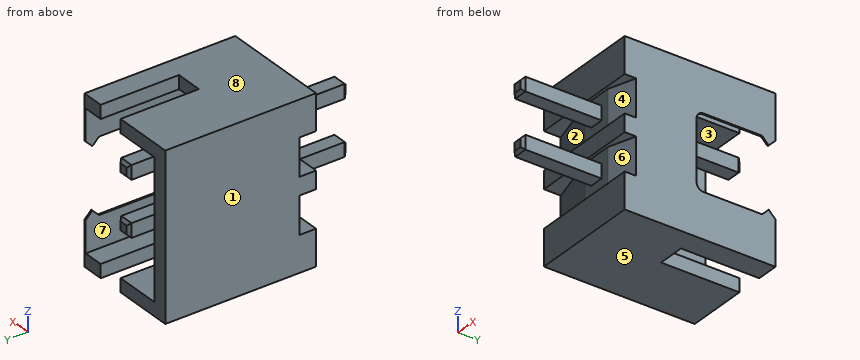
```python
from build123d import *

# Parameters (mm, degrees)
SKETCH1_W           = 6.8453
SKETCH1_H           = 7.4295
BOSS_EXTRUDE1_DEPTH = 5
SKETCH2_W           = 5.8039
SKETCH2_H           = 0.127
CUT_EXTRUDE1_DEPTH  = 5.7277
CUT_EXTRUDE2_DEPTH  = 1.6891
CUT_EXTRUDE3_DEPTH  = 1.6891
SKETCH5_W           = 5
SKETCH5_H           = 4.1148
BOSS_EXTRUDE2_DEPTH = 0.127
SKETCH6_W           = 3.3147
SKETCH6_H           = 0.127
CUT_EXTRUDE4_DEPTH  = 6
CUT_EXTRUDE5_DEPTH  = 1.6891
CUT_EXTRUDE6_DEPTH  = 1.6891
SKETCH9_W           = 5
SKETCH9_H           = 1.6256
BOSS_EXTRUDE3_DEPTH = 0.127
SKETCH10_W          = 4.2672
SKETCH10_H          = 6.2103
CUT_EXTRUDE7_DEPTH  = 5.1308
CUT_EXTRUDE8_DEPTH  = 1.0724
SKETCH12_W          = 1.2319
SKETCH12_H          = 3.556
CUT_EXTRUDE9_DEPTH  = 1.6096
SKETCH13_W          = 1.2319
SKETCH13_H          = 3.556
CUT_EXTRUDE10_DEPTH = 8.4295
SKETCH14_W          = 0.635
SKETCH14_H          = 0.635
BOSS_EXTRUDE4_DEPTH = 3.5814
SKETCH15_W          = 0.635
SKETCH15_H          = 0.635
BOSS_EXTRUDE5_DEPTH = 3.5814
SKETCH16_W          = 0.635
SKETCH16_H          = 0.635
BOSS_EXTRUDE6_DEPTH = 4.7625
SKETCH17_W          = 0.635
SKETCH17_H          = 0.635
BOSS_EXTRUDE7_DEPTH = 4.7625
DRAFT1_ANGLE        = 45
DRAFT2_ANGLE        = 45
CHAMFER1_SIZE       = 0.127
FILLET1_R           = 0.3175


with BuildPart() as part:
    # Sketch1 → Boss-Extrude1 (new body)
    with BuildSketch(Plane(origin=(-5.7277, 0, 0), x_dir=(0, -1, 0), z_dir=(-1, 0, 0))):
        with Locations((-3.42265, -3.71475)):
            Rectangle(SKETCH1_W, SKETCH1_H)
    extrude(amount=-BOSS_EXTRUDE1_DEPTH)

    # Sketch2 → Cut-Extrude1 (cut)
    with BuildSketch(Plane.ZY.offset(5.7277)):
        with Locations((-4.52755, 0.0635)):
            Rectangle(SKETCH2_W, SKETCH2_H)
    extrude(amount=-CUT_EXTRUDE1_DEPTH, mode=Mode.SUBTRACT)

    # Sketch3 → Cut-Extrude2 (cut)
    with BuildSketch(Plane.XY.offset(-1.6256)):
        Polygon((-5.7277, 0.127), (-3.3477, 0.127), (-5.7277, 0.762), align=None)
    extrude(amount=-CUT_EXTRUDE2_DEPTH, mode=Mode.SUBTRACT)

    # Sketch4 → Cut-Extrude3 (cut)
    with BuildSketch(Plane.XY.offset(-1.6256)):
        Polygon((-1.94, 0.127), (0, 0.127), (0, 0.762), align=None)
    extrude(amount=-CUT_EXTRUDE3_DEPTH, mode=Mode.SUBTRACT)

    # Sketch5 → Boss-Extrude2 (add)
    with BuildSketch(Plane.XZ.offset(-0.127)):
        with Locations((-3.2277, -5.3721)):
            Rectangle(SKETCH5_W, SKETCH5_H)
    extrude(amount=BOSS_EXTRUDE2_DEPTH)

    # Sketch6 → Cut-Extrude4 (cut, through all)
    with BuildSketch(Plane.ZY.offset(5.7277)):
        with Locations((-5.77215, 0.0635)):
            Rectangle(SKETCH6_W, SKETCH6_H)
    extrude(amount=-CUT_EXTRUDE4_DEPTH, mode=Mode.SUBTRACT)

    # Sketch7 → Cut-Extrude5 (cut)
    with BuildSketch(Plane.XY.offset(-4.1148)):
        Polygon((-5.7277, 0.127), (-3.3477, 0.127), (-5.7277, 0.762), align=None)
    extrude(amount=-CUT_EXTRUDE5_DEPTH, mode=Mode.SUBTRACT)

    # Sketch8 → Cut-Extrude6 (cut)
    with BuildSketch(Plane.XY.offset(-4.1148)):
        Polygon((-1.94, 0.127), (0, 0.127), (0, 0.762), align=None)
    extrude(amount=-CUT_EXTRUDE6_DEPTH, mode=Mode.SUBTRACT)

    # Sketch9 → Boss-Extrude3 (add)
    with BuildSketch(Plane.XZ.offset(-0.127)):
        with Locations((-3.2277, -6.6167)):
            Rectangle(SKETCH9_W, SKETCH9_H)
    extrude(amount=BOSS_EXTRUDE3_DEPTH)

    # Sketch10 → Cut-Extrude7 (cut)
    with BuildSketch(Plane(origin=(0, 6.8453, 0), x_dir=(-1, 0, 0), z_dir=(0, 1, 0))):
        with Locations((2.9337, -3.71475)):
            Rectangle(SKETCH10_W, SKETCH10_H)
    extrude(amount=-CUT_EXTRUDE7_DEPTH, mode=Mode.SUBTRACT)

    # Sketch11 → Cut-Extrude8 (cut, through all)
    with BuildSketch(Plane.ZY.offset(0.8001)):
        Polygon((-2.032, 6.8453), (-5.3975, 6.8453), (-4.7879, 6.2357), (-5.3975, 6.2357), (-5.3975, 3.2639), (-2.032, 3.2639), (-2.032, 6.2357), (-2.6416, 6.2357), align=None)
    extrude(amount=-CUT_EXTRUDE8_DEPTH, mode=Mode.SUBTRACT)

    # Sketch12 → Cut-Extrude9 (cut, through all)
    with BuildSketch(Plane(origin=(0, 0, -0.6096), x_dir=(-1, 0, 0), z_dir=(0, 0, -1))):
        with Locations((2.34365, 5.0673)):
            Rectangle(SKETCH12_W, SKETCH12_H)
    extrude(amount=-CUT_EXTRUDE9_DEPTH, mode=Mode.SUBTRACT)

    # Sketch13 → Cut-Extrude10 (cut, through all)
    with BuildSketch(Plane(origin=(0, 0, -7.4295), x_dir=(-1, 0, 0), z_dir=(0, 0, -1))):
        with Locations((2.34365, 5.0673)):
            Rectangle(SKETCH13_W, SKETCH13_H)
    extrude(amount=-CUT_EXTRUDE10_DEPTH, mode=Mode.SUBTRACT)

    # Sketch14 → Boss-Extrude4 (add)
    with BuildSketch(Plane.XZ.offset(-0.127)):
        with Locations((-2.6452, -4.95935)):
            Rectangle(SKETCH14_W, SKETCH14_H)
    extrude(amount=BOSS_EXTRUDE4_DEPTH)

    # Sketch15 → Boss-Extrude5 (add)
    with BuildSketch(Plane.XZ.offset(-0.127)):
        with Locations((-2.6452, -2.47015)):
            Rectangle(SKETCH15_W, SKETCH15_H)
    extrude(amount=BOSS_EXTRUDE5_DEPTH)

    # Sketch16 → Boss-Extrude6 (add)
    with BuildSketch(Plane(origin=(0, 1.7145, 0), x_dir=(-1, 0, 0), z_dir=(0, 1, 0))):
        with Locations((2.6452, -4.95935)):
            Rectangle(SKETCH16_W, SKETCH16_H)
    extrude(amount=BOSS_EXTRUDE6_DEPTH)

    # Sketch17 → Boss-Extrude7 (add)
    with BuildSketch(Plane(origin=(0, 1.7145, 0), x_dir=(-1, 0, 0), z_dir=(0, 1, 0))):
        with Locations((2.6452, -2.47015)):
            Rectangle(SKETCH17_W, SKETCH17_H)
    extrude(amount=BOSS_EXTRUDE7_DEPTH)

    # Draft1
    draft1_faces = [part.faces().sort_by_distance(p)[0] for p in [
        (-0.7639, 6.2357, -2.3368),
    ]]
    draft(draft1_faces, Plane(origin=(-0.7277, 3.2639, -2.032), x_dir=(-1, 0, 0), z_dir=(0, 0, -1)), DRAFT1_ANGLE)

    # Draft2
    draft2_faces = [part.faces().sort_by_distance(p)[0] for p in [
        (-0.7639, 6.2357, -5.0927),
    ]]
    draft(draft2_faces, Plane(origin=(-0.7277, 6.2357, -5.3975), x_dir=(1, 0, 0), z_dir=(0, 0, 1)), DRAFT2_ANGLE)

    # Chamfer1
    chamfer1_edges = [part.edges().sort_by_distance(p)[0] for p in [
        (-2.3277, -3.4544, -4.95935),
        (-2.6452, -3.4544, -4.64185),
        (-2.9627, -3.4544, -4.95935),
        (-2.6452, -3.4544, -5.27685),
        (-2.9627, -3.4544, -2.47015),
        (-2.6452, -3.4544, -2.78765),
        (-2.3277, -3.4544, -2.47015),
        (-2.6452, -3.4544, -2.15265),
        (-2.6452, 6.477, -4.64185),
        (-2.3277, 6.477, -4.95935),
        (-2.6452, 6.477, -5.27685),
        (-2.9627, 6.477, -4.95935),
        (-2.3277, 6.477, -2.47015),
        (-2.6452, 6.477, -2.78765),
        (-2.9627, 6.477, -2.47015),
        (-2.6452, 6.477, -2.15265),
    ]]
    chamfer(chamfer1_edges, length=CHAMFER1_SIZE)

    # Fillet1
    fillet1_edges = [part.edges().sort_by_distance(p)[0] for p in [
        (-0.7639, 3.2639, -2.032),
        (-0.7639, 3.2639, -5.3975),
    ]]
    fillet(fillet1_edges, radius=FILLET1_R)


solid = part.part
```
For this review, take the finished solid that the model builds, in its own axes (mm). Face numbers are marked on the shaded views. A direction names the side the tool comes from. Coordinates: 2 decimals unless noted, no trailing zeros. Write each loop counter-clockwise with the first axis right and the second up, starting at its lowest first coordinate (ties: lowest second). Pieces come first, ordered by that corner, then holes.
(1) Tool access review of the marked faces 1, 2, 3, 4 and 5: name each direction out of +Z, -Z, +X, -X, +Y, -Y from which nothing blocks a thin tool from reaching the whole face with its end or side.
(2) Add section A-A on y = -2. Give the boundary of the cut face in (x, z).
(3) Wall thickness on probe 1 along Z at (x, y) = (-4.35, 0.25); probe 2 along Z at (x, y) = (-3.05, 4.75); probe 3 along X at (y, z) = (6.75, -0.5): over which ranges is each line inside the solid? List them lowest first.
(4) Add section B-B on z = -0.5. Give the boundary of the cut face in (x, y), then the cut area to 3 significant figures.
(5) Add section D-D on x = -4.05. Give the boundary of the cut face in (y, z).
(6) For pin 1 Ø1.8 at (x, z) = (-4, -1) entering from -Y; pin 2 Ø0.5 at (y, z) = (4.5, -2.5) entering from +X; pin 3 Ø0.5 at (y, z) = (-2, -2.5) entering from -X, all flat-tipped, find the tip position at first contact; note any pin that passes through.
(7) The part is to be moulded in two halves that separate along X. For the marked faces 6, 7 and 8, say which applies: +X half, -X half, draft (parallel to the pull), parting line (faces both ways), or undercut.
(8) Add section C-C on y = 4.5. Give the boundary of the cut face in (x, z), then the cut area to 3 significant figures.
Answer sheet:
1. face 1: +Z, -Z, -X, +Y, -Y
1. face 2: -X, -Y
1. face 3: +Y
1. face 4: +X, -Y
1. face 5: -Z, +X, -X, +Y, -Y
2. outline: (-2.96, -5.28) - (-2.33, -5.28) - (-2.33, -4.64) - (-2.96, -4.64) - close; (-2.96, -2.79) - (-2.33, -2.79) - (-2.33, -2.15) - (-2.96, -2.15) - close
3. probe 1: z = -7.43 to -5.8, -4.11 to -3.31, -1.63 to 0
3. probe 2: z = -7.43 to -6.82, -0.61 to 0
3. probe 3: x = -5.73 to -2.96, -1.73 to -0.73
4. outline: (-5.73, 0) - (-0.73, 0) - (-0.73, 6.85) - (-1.73, 6.85) - (-1.73, 3.29) - (-2.96, 3.29) - (-2.96, 6.85) - (-5.73, 6.85) - close
4. area: 29.8 mm2
5. outline: (0, -7.43) - (6.85, -7.43) - (6.85, -6.82) - (1.71, -6.82) - (1.71, -0.61) - (6.85, -0.61) - (6.85, 0) - (0, 0) - (0, -1.63) - (0.31, -1.63) - (0.31, -3.31) - (0, -3.31) - (0, -4.11) - (0.31, -4.11) - (0.31, -5.8) - (0, -5.8) - close
6. pin 1: stops at y = 0
6. pin 2: stops at x = -2.33
6. pin 3: stops at x = -2.96
7. face 6: +X half
7. face 7: undercut
7. face 8: draft
8. outline: (-5.73, -7.43) - (-2.96, -7.43) - (-2.96, -6.82) - (-5.07, -6.82) - (-5.07, -0.61) - (-2.96, -0.61) - (-2.96, 0) - (-5.73, 0) - close; (-2.96, -5.28) - (-2.33, -5.28) - (-2.33, -4.64) - (-2.96, -4.64) - close; (-2.96, -2.79) - (-2.33, -2.79) - (-2.33, -2.15) - (-2.96, -2.15) - close; (-1.73, -7.43) - (-0.73, -7.43) - (-0.73, -5.4) - (-0.8, -5.4) - (-0.8, -6.82) - (-1.73, -6.82) - close; (-1.73, -0.61) - (-0.8, -0.61) - (-0.8, -2.03) - (-0.73, -2.03) - (-0.73, 0) - (-1.73, 0) - close
8. area: 9.71 mm2
